Part model, mm, in its own coordinate system. Face numbers are marked on the shaded views. A direction names the side the tool comes from. Round coordinates to 2 decimals unless told otherwise and drop trailing zeros. Write each loop counter-clockwise with the first axis right and the second up, starting at its lowest first coordinate (ties: lowest second). Pieces come first, ordered by that corner, then holes.
```python
from build123d import *

# Parameters (mm, degrees)
SKETCH1_W               = 13
SKETCH1_H               = 13
BOSS_EXTRUDE1_DEPTH     = 5
SKETCH2_W               = 13
SKETCH2_H               = 5
BOSS_EXTRUDE2_DEPTH     = 16.4
SKETCH3_W               = 13
SKETCH3_H               = 10
BOSS_EXTRUDE3_DEPTH     = 17.6
SKETCH4_R               = 8.25
CUT_EXTRUDE1_DEPTH      = 13
SKETCH5_W               = 13
SKETCH5_H               = 22.6
BOSS_EXTRUDE4_DEPTH     = 3.25
CUT_EXTRUDE2_DEPTH      = 1
CUT_EXTRUDE2_DEPTH_BACK = 1
CUT_EXTRUDE2_START      = -2.5
CUT_EXTRUDE3_REACH      = 37.169
FILLET2_R               = 2


with BuildPart() as part:
    # Sketch1 → Boss-Extrude1 (new body)
    with BuildSketch(Plane(origin=(0, 0, 0), x_dir=(1, 0, 0), z_dir=(0, 1, 0))):
        Rectangle(SKETCH1_W, SKETCH1_H)
    extrude(amount=BOSS_EXTRUDE1_DEPTH)

    # Sketch2 → Boss-Extrude2 (add)
    with BuildSketch(Plane(origin=(0, 0, -6.5), x_dir=(-1, 0, 0), z_dir=(0, 0, -1))):
        with Locations((0, 2.5)):
            Rectangle(SKETCH2_W, SKETCH2_H)
    extrude(amount=BOSS_EXTRUDE2_DEPTH)

    # Sketch3 → Boss-Extrude3 (add)
    with BuildSketch(Plane(origin=(0, 5, 0), x_dir=(1, 0, 0), z_dir=(0, 1, 0))):
        with Locations((0, 17.9)):
            Rectangle(SKETCH3_W, SKETCH3_H)
    extrude(amount=BOSS_EXTRUDE3_DEPTH)

    # Sketch4 → Cut-Extrude1 (cut)
    with BuildSketch(Plane(origin=(6.5, 0, 0), x_dir=(0, 0, -1), z_dir=(1, 0, 0))):
        with Locations((12.9, 13.8)):
            Circle(SKETCH4_R)
    extrude(amount=-CUT_EXTRUDE1_DEPTH, mode=Mode.SUBTRACT)

    # Sketch5 → Boss-Extrude4 (add)
    with BuildSketch(Plane(origin=(0, 0, -22.9), x_dir=(-1, 0, 0), z_dir=(0, 0, -1))):
        with Locations((0, 11.3)):
            Rectangle(SKETCH5_W, SKETCH5_H)
    extrude(amount=BOSS_EXTRUDE4_DEPTH)

    # Sketch6 → Cut-Extrude2 (cut, two sides: drawn at the far end of the back side and taken through both)
    with BuildSketch(Plane.XZ.offset(CUT_EXTRUDE2_START - CUT_EXTRUDE2_DEPTH_BACK)):
        Polygon((5.65, 2.258696921), (5.65, -26.15), (1.35, -26.15), (1.35, 2.258696921), (1.35, 4.741303079), (3.5, 5.982606158), (5.65, 4.741303079), align=None)
        Polygon((-1.35, 2.258696921), (-1.35, 4.741303079), (-3.5, 5.982606158), (-5.65, 4.741303079), (-5.65, 2.258696921), (-5.65, -26.15), (-1.35, -26.15), align=None)
    extrude(amount=CUT_EXTRUDE2_DEPTH + CUT_EXTRUDE2_DEPTH_BACK, mode=Mode.SUBTRACT)

    # Cut-Extrude3: up to this face of the body (flat: up to its plane)
    cut_extrude3_end = Plane(part.part.faces().sort_by_distance((0, 5, -3.2))[0])
    # Sketch7 → Cut-Extrude3 (cut, up to the picked face)
    with BuildSketch(Plane.XZ, mode=Mode.PRIVATE) as cut_extrude3_sk1:
        with BuildLine():
            Line((-2.3, 3.5), (-2.3, -9.5))
            Line((-2.3, -9.5), (-4.7, -9.5))
            Line((-4.7, -9.5), (-4.7, 3.5))
            ThreePointArc((-4.7, 3.5), (-3.5, 4.7), (-2.3, 3.5))
        make_face()
    cut_extrude3_tool1 = split(extrude(cut_extrude3_sk1.sketch, amount=-CUT_EXTRUDE3_REACH, mode=Mode.PRIVATE), bisect_by=cut_extrude3_end, keep=Keep.BOTH, mode=Mode.PRIVATE)
    # Sketch7 → Cut-Extrude3 (cut, up to the picked face)
    with BuildSketch(Plane.XZ, mode=Mode.PRIVATE) as cut_extrude3_sk2:
        with BuildLine():
            Line((2.3, 3.5), (2.3, -9.5))
            Line((2.3, -9.5), (4.7, -9.5))
            Line((4.7, -9.5), (4.7, 3.5))
            ThreePointArc((4.7, 3.5), (3.5, 4.7), (2.3, 3.5))
        make_face()
    cut_extrude3_tool2 = split(extrude(cut_extrude3_sk2.sketch, amount=-CUT_EXTRUDE3_REACH, mode=Mode.PRIVATE), bisect_by=cut_extrude3_end, keep=Keep.BOTH, mode=Mode.PRIVATE)
    add(cut_extrude3_tool1.solids().sort_by(Axis((-3.5, 0, -2.526189), (0, 1, 0)))[0], mode=Mode.SUBTRACT)
    add(cut_extrude3_tool2.solids().sort_by(Axis((3.5, 0, -2.526189), (0, 1, 0)))[0], mode=Mode.SUBTRACT)

    # Fillet2
    # the kernel refuses this fillet: 2 mm, written as the material it takes off along each edge
    with BuildSketch(Plane(origin=(-11.5, 0, 6.5), x_dir=(0, 1, 0), z_dir=(1, 0, 0)), Plane(origin=(-11.5, 0, -26.15), x_dir=(0, 0, 1), z_dir=(1, 0, 0))) as fillet2_piece_1:
        with BuildLine():
            CenterArc((FILLET2_R, -FILLET2_R), FILLET2_R, 90, 90)
            Line((0, -FILLET2_R), (0, 0))
            Line((0, 0), (FILLET2_R, 0))
        make_face()
    extrude(amount=23, mode=Mode.SUBTRACT)
    with BuildSketch(Plane(origin=(-11.5, 5, 6.5), x_dir=(0, -1, 0), z_dir=(1, 0, 0)), Plane(origin=(11.5, 22.6, -26.15), x_dir=(0, -1, 0), z_dir=(-1, 0, 0))) as fillet2_piece_2:
        with BuildLine():
            CenterArc((FILLET2_R, FILLET2_R), FILLET2_R, 180, 90)
            Line((0, FILLET2_R), (0, 0))
            Line((0, 0), (FILLET2_R, 0))
        make_face()
    extrude(amount=23, mode=Mode.SUBTRACT)
    with BuildSketch(Plane(origin=(-9.491448846, 5.55, -12.9), x_dir=(0, 0.0725199720178057, -0.9973669603804493), z_dir=(1, 0, 0))) as fillet2_piece_3:
        with BuildLine():
            CenterArc((1.341619482, -1.994733921), FILLET2_R, 94.15873901, 39.530984807)
            Line((-0.039885985, -0.548551828), (0, 0))
            ThreePointArc((0, 0), (0.598289769, -0.021722577), (1.196579538, 0))
        make_face()
    extrude(amount=18.982897691, mode=Mode.SUBTRACT)
    with BuildSketch(Plane(origin=(-9.491448846, 22.05, -12.9), x_dir=(0, 1, 0), z_dir=(1, 0, 0))) as fillet2_piece_4:
        with BuildLine():
            CenterArc((1.8921875, -1.482744993), FILLET2_R, 132.151537174, 39.530984807)
            ThreePointArc((-0.086775915, -1.193428897), (-0.021722577, -0.598289769), (0, 0))
            Line((0, 0), (0.55, 0))
        make_face()
    extrude(amount=18.982897691, mode=Mode.SUBTRACT)


solid = part.part
```
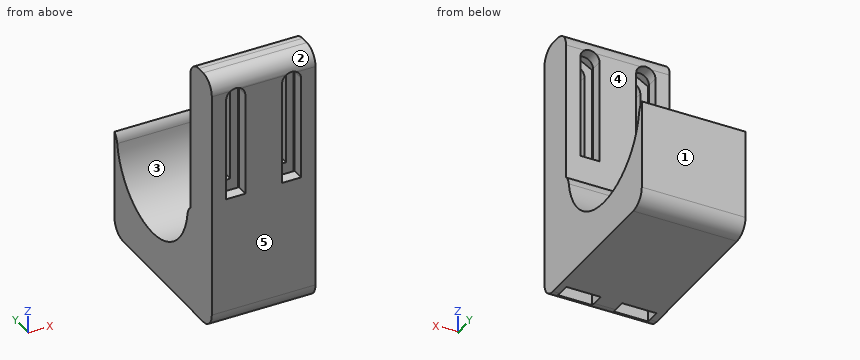
Q1. Which spindle directions (+Z, -Z, +X, -X, +Y, -Y) get a long thin tool onto all of the face, cutting with end or side? Do the marked faces 4 and 5. Say none if no direction does.
Values follow:
face 4: +Z, +X, -X, +Y
face 5: +Z, -Z, +X, -X, -Y
Q2. Cut at A-A on z = -9. Write the cut outline in (x, y), plus the area to 3 significant figures.
Values follow:
outline: (-6.5, 0) - (-4.7, 0) - (-4.7, 1.5) - (-5.65, 1.5) - (-5.65, 3.5) - (-4.7, 3.5) - (-4.7, 5) - (-6.5, 5) - close; (-2.3, 0) - (2.3, 0) - (2.3, 1.5) - (1.35, 1.5) - (1.35, 3.5) - (2.3, 3.5) - (2.3, 5) - (-2.3, 5) - (-2.3, 3.5) - (-1.35, 3.5) - (-1.35, 1.5) - (-2.3, 1.5) - close; (4.7, 0) - (6.5, 0) - (6.5, 5) - (4.7, 5) - (4.7, 3.5) - (5.65, 3.5) - (5.65, 1.5) - (4.7, 1.5) - close
area: 33.4 mm2
Q3. Mould opens along Y. For the marked faces 1, 2 and 3 say: +Y half, -Y half, draft (parallel to the pull), parting line (faces both ways), or undercut.
Values follow:
face 1: +Y half
face 2: -Y half
face 3: undercut
Q4. Drop flat-ended pins along their axis: pin 1 (1 mm diameter, centred on x = 0, z = -13, fed in from -Y); pin 2 (0.8 mm diameter, centred on x = 4, y = 4, fed in from +Z); pin 3 (4.5 mm diameter, centred on x = -4, z = -3, fed in from +Y); pin 4 (1.2 mm diameter, centred on x = -3.5, y = 1, fed in from +Z). Give the stop position or say it passes through.
Values follow:
pin 1: stops at y = 0
pin 2: stops at z = 6.41
pin 3: stops at y = 5
pin 4: stops at z = 6.46
Q5. Wall check: L1, parallel to X at y = 2, z = -6.5; L2, parallel to Y at x = 2.5, z = -10; L3, parallel to Y at x = -4.5, z = -24. Give the ranges that are in metal, low to high.
Values follow:
L1: x = -6.5 to -5.65, -1.35 to 1.35, 5.65 to 6.5
L2: y = 0 to 1.5, 3.5 to 5
L3: y = 0 to 1.5, 3.5 to 22.6
Q6. Cut at B-B on x = -0.75. Write the cut outline in (y, z), plus the area to 3 significant figures.
Values follow:
outline: (0, -24.15) arc R2 ccw to (2, -26.15) - (20.6, -26.15) arc R2 ccw to (22.6, -24.15) - (22.6, -12.9) arc R2 ccw to (21.96, -14.09) arc R8.25 cw to (5.64, -14.09) arc R2 ccw to (5, -12.9) - (5, 4.5) arc R2 ccw to (3, 6.5) - (2, 6.5) arc R2 ccw to (0, 4.5) - close
area: 286 mm2
Q7. Cut at D-D on x = 1.75. Write the cut outline in (y, z).
Values follow:
outline: (0, -24.15) arc R2 ccw to (1.5, -26.09) - (1.5, 4.97) - (3.5, 4.97) - (3.5, -26.15) - (20.6, -26.15) arc R2 ccw to (22.6, -24.15) - (22.6, -12.9) arc R2 ccw to (21.96, -14.09) arc R8.25 cw to (5.64, -14.09) arc R2 ccw to (5, -12.9) - (5, 4.5) arc R2 ccw to (3, 6.5) - (2, 6.5) arc R2 ccw to (0, 4.5) - close
Q8. Cut at C-C on y = 19. Write the cut outline in (x, z).
Values follow:
outline: (-6.5, -26.15) - (6.5, -26.15) - (6.5, -19.3) - (-6.5, -19.3) - close
